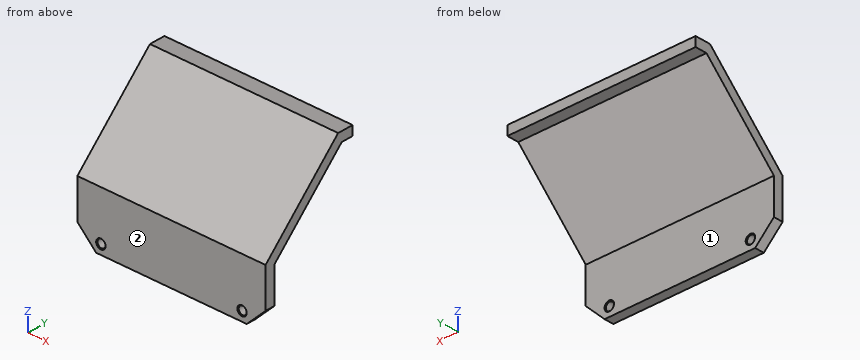
Solid Edge part; units mm, degrees
sketch "Sketch1" plane through (0, 0, 0) normal (1, 0, 0) x (0, 1, 0)
  line L0 (0, 0) -> (4, 0)
  line L1 (4, 0) -> (4, 15)
  line L2 (4, 15) -> (35, 46)
  line L3 (35, 46) -> (40, 46)
  line L4 (40, 46) -> (40, 50)
  line L5 (40, 50) -> (33.3431, 50)
  line L6 (33.3431, 50) -> (0, 16.6569)
  line L7 (0, 16.6569) -> (0, 0)
  dimension "D1" = 4
extrude "Protrusion1" add sketch "Sketch1" along normal mid plane 80
sketch "Sketch2" plane through (0, 0, 8.3284) normal (0, -1, 0) x (1, 0, 0)
  line L0 (-40, -8.3284) -> (40, -8.3284)
  line L1 (40, -8.3284) -> (32, -16.3284)
  line L2 (32, -16.3284) -> (-32, -16.3284)
  line L3 (-32, -16.3284) -> (-40, -8.3284)
  dimension "D1" = 40
  dimension "D2" = 40
  dimension "D3" = 32
extrude "Protrusion2" add sketch "Sketch2" against normal up to vertex (4 mm away)
hole "Hole1" at (-30, 0, -4) direction (0, 1, 0) diameter 3.4 end up to next start chamfer 0.3 start chamfer angle 45 end chamfer 0.3 end chamfer angle 45
hole "Hole2" at (30, 0, -4) direction (0, 1, 0) diameter 3.4 end up to next start chamfer 0.3 start chamfer angle 45 end chamfer 0.3 end chamfer angle 45
properties material "Polyethylene, low density"
CAD build for the part. Positions are in the model's coordinates, mm. Face numbers are marked on the shaded views. A direction names the side the tool comes from. Round coordinates to 2 decimals unless told otherwise and drop trailing zeros. Loops run counter-clockwise (first coordinate to the right, second up) from the corner with the lowest first, then second, coordinate; pieces in that order, holes last. Notation, with made-up numbers: M 0,16 L 24,16 A18 cw 24,24 Z; hole C 65.5,20.25 d10. An arc over 180 degrees is marked long. Return JSON: item names as keys, results as strings. Group by question number.
(1) Saw through at C-C, the plane z = 12.5. List the corners of the cut face in (x, y), and give its area (3 significant figures).
(2) Tool access for the marked faces 1 and 2: list every direction of +Z, -Z, +X, -X, +Y, -Y with a clear straight run to the whole face (end or side of a thin tool).
(3) Saw through at B-B, the plane x = -30. List the corners of the cut face in (y, z), and give its area (3 significant figures).
(4) Saw through at A-A, the plane z = -4. List the corners of the cut face in (x, y), and give its area (3 significant figures).
(5) Wall check: probe 1 along X at (y, z) = (2, -4); probe 2 along Z at (x, y) = (0, 35.5); probe 3 along Y at (x, z) = (34.5, 7.5). Give the ranges that are in metal, low to high. Write a range as [from, to].
(6) Drop flat-ended pins along their axis: P1, Ø1, axis at x = -26.5, y = 19, coming from the -Z side; P2, Ø4, axis at x = 0.5, z = 26, coming from the -Y side; P3, Ø6, axis at x = -27.5, y = 21.5, coming from the +Z side. Give the stop position or say it passes through.
(7) Saw through at D-D, the plane y = 26. List the corners of the cut face in (x, z).
Answer list:
{
 "1": {"outline": "M -40,0 L 40,0 L 40,4 L -40,4 Z", "area": "320 mm2"},
 "2": {"face 1": "-Z, +X, -X, +Y", "face 2": "+Z, -Z, +X, -X, -Y"},
 "3": {"outline": "M 0,-8 L 4,-8 L 4,-6 L 3.7,-5.7 L 0.3,-5.7 L 0,-6 Z; M 0,-2 L 0.3,-2.3 L 3.7,-2.3 L 4,-2 L 4,15 L 35,46 L 40,46 L 40,50 L 33.34,50 L 0,16.66 Z", "area": "287 mm2"},
 "4": {"outline": "M -36,0 L -32,0 L -31.7,0.3 L -31.7,3.7 L -32,4 L -36,4 Z; M -28.3,0.3 L -28,0 L 28,0 L 28.3,0.3 L 28.3,3.7 L 28,4 L -28,4 L -28.3,3.7 Z; M 31.7,0.3 L 32,0 L 36,0 L 36,4 L 32,4 L 31.7,3.7 Z", "area": "260 mm2"},
 "5": {"probe 1": "[-36, -31.7], [-28.3, 28.3], [31.7, 36]", "probe 2": "[46, 50]", "probe 3": "[0, 4]"},
 "6": {"P1": "z = 29.5", "P2": "y = 7.34", "P3": "z = 41.16"},
 "7": {"outline": "M -40,37 L 40,37 L 40,42.66 L -40,42.66 Z"}
}
